The model under review builds one solid part; all positions refer to its coordinate system, in mm. A direction names the side the tool comes from. Give positions to 0.01 mm unless a question says otherwise; leave off trailing zeros. Loops run counter-clockwise (first coordinate to the right, second up) from the corner with the lowest first, then second, coordinate; pieces in that order, holes last. Notation, with made-up numbers: (79, 46.25) -> (108, 46.25) arc R23 cw to (108, 67.25) -> close; hole circle Ø4 at (34, -1). An arc over 180 degrees is marked (long way). Write each question's results on one line, items separated by ' | '. Start each with the question number.
Q1. Mouldability with a two-part tool opening along X and no side actions: class faces 1 (the face through (0, 127, 9)), 2 (the face through (6.35, 64, 16)), 3 (the face through (-0.18, 70.13, 15.9)), 4 (the face through (-6.35, 64, 16)) as released by +X, released by -X, zero draft, split by the parting line, or undercut.
Q2. Insertion check: pin 1 Ø6 at (x, y) = (0, 69.85) entering from +Z. The pin has a flat end and moves straight along its axis. Give the tip position at first contact, or say it passes through.
Q3. We need section B-B (y = 73). Write out the cut boundary in (x, z), plus the area to 3 significant figures.
Q4. We need section A-A (x = -3). Write out the cut boundary in (y, z).
Q5. We need section C-C (z = 39.5). Write out the cut boundary in (x, y).
Q6. Machinability: for faces 5 (the face through (0, 63, 0)), 6 (the face through (-0.412, 67.996, 7.585)), which of the approach directions +Z, -Z, +X, -X, +Y, -Y give a long, thin tool a straight path to every point of the face, cutting with its end or side? Answer none if there is none.
Q7. Wall thickness on L1, parallel to Y at x = 0, z = 8.25; L2, parallel to X at y = 69.85, z = 8; L3, parallel to Y at x = -1.5, z = 11: over which ranges is each line inside the solid? List them lowest first. Write a range as [from, to].
from build123d import *

# Parameters (mm, degrees)
BOSS_EXTRUDE1_DEPTH        = 6.35
F_10_24_TAPPED_HOLE1_D     = 3.7973
F_10_24_TAPPED_HOLE1_DEPTH = 14.9606
F_10_24_TAPPED_HOLE1_TIP   = 1.140824014
FILLET1_R                  = 12.7


with BuildPart() as part:
    # Sketch1 → Boss-Extrude1 (new, symmetric)
    with BuildSketch(Plane(origin=(0, 0, 0), x_dir=(0, 0, -1), z_dir=(1, 0, 0))):
        with BuildLine():
            Line((0, 0), (0, 127))
            Line((0, 127), (-29.89679252, 127))
            Line((-29.89679252, 127), (-41.522242414, 6.962121916))
            ThreePointArc((-41.522242414, 6.962121916), (-39.903382192, 2.08177286), (-35.201814678, 0))
            Line((-35.201814678, 0), (0, 0))
        make_face()
    extrude(amount=BOSS_EXTRUDE1_DEPTH, both=True)

    # #10-24 Tapped Hole1
    with Locations(Plane(origin=(0, 0, 0), x_dir=(-1, 0, 0), z_dir=(0, 0, -1))):
        with Locations((0, 12.7), (0, 69.85)):
            Hole(F_10_24_TAPPED_HOLE1_D / 2, depth=F_10_24_TAPPED_HOLE1_DEPTH)
            with Locations((0, 0, -(F_10_24_TAPPED_HOLE1_DEPTH + F_10_24_TAPPED_HOLE1_TIP / 2))):  # 118° drill point
                Cone(0, F_10_24_TAPPED_HOLE1_D / 2, F_10_24_TAPPED_HOLE1_TIP, mode=Mode.SUBTRACT)

    # Fillet1
    fillet1_edges = [part.edges().sort_by_distance(p)[0] for p in [
        (0, 127, 29.89679252),
    ]]
    fillet(fillet1_edges, radius=FILLET1_R)


solid = part.part
Output:
1) face 1: zero draft | face 2: released by +X | face 3: undercut | face 4: released by -X
2) pin 1: z = 35.72
3) outline: (-6.35, 0) -> (6.35, 0) -> (6.35, 35.13) -> (-6.35, 35.13) -> close | area: 446 mm2
4) outline: (0, 0) -> (127, 0) -> (127, 18.37) arc R12.7 ccw to (115.52, 31.01) -> (6.96, 41.52) arc R6.35 ccw to (0, 35.2) -> close
5) outline: (-6.35, 1.68) -> (6.35, 1.68) -> (6.35, 27.84) -> (-6.35, 27.84) -> close
6) face 5: -Z, +X, -X, +Y, -Y | face 6: -Z
7) L1: [0, 10.8], [14.6, 67.95], [71.75, 127] | L2: [-6.35, -1.9], [1.9, 6.35] | L3: [0, 11.54], [13.86, 68.69], [71.01, 127]
